from build123d import *

# Parameters (mm, degrees)
SKETCH_1_W          = 75
SKETCH_1_H          = 75
EXTRUDE_1_DEPTH     = 84
CHAMFER_1_SIZE      = 3
SKETCH_2_R          = 4.25
CUT_EXTRUDE_1_DEPTH = 85


with BuildPart() as part:
    # 草图1 → 凸台-拉伸1 (new body)
    with BuildSketch(Plane.XY):
        with Locations((37.5, -37.5)):
            Rectangle(SKETCH_1_W, SKETCH_1_H)
    extrude(amount=EXTRUDE_1_DEPTH)

    # 倒角1
    chamfer_1_edges = [part.edges().sort_by_distance(p)[0] for p in [
        (0, 0, 42),
        (75, 0, 42),
        (75, -75, 42),
        (0, -75, 42),
    ]]
    chamfer(chamfer_1_edges, length=CHAMFER_1_SIZE)

    # 草图2 → 切除-拉伸1 (cut, through all)
    with BuildSketch(Plane.XY.offset(84)):
        with Locations((7.5, -7.5)):
            Circle(SKETCH_2_R)
        with Locations((67.5, -7.5)):
            Circle(SKETCH_2_R)
        with Locations((67.5, -67.5)):
            Circle(SKETCH_2_R)
        with Locations((7.5, -67.5)):
            Circle(SKETCH_2_R)
    extrude(amount=-CUT_EXTRUDE_1_DEPTH, mode=Mode.SUBTRACT)


solid = part.part
Source: CAD feature listing. Evaluate the final solid. Frame: model axes, mm. Round coordinates to 2 decimals unless told otherwise and drop trailing zeros. Loops run counter-clockwise (first coordinate to the right, second up) from the corner with the lowest first, then second, coordinate; pieces in that order, holes last. Notation, with made-up numbers: (6.5, 68) -> (33.5, 68) arc R35 cw to (33.5, 100) -> close; hole circle Ø10 at (-32.5, 82). An arc over 180 degrees is marked (long way). Answer as a JSON object with one key per item and string values. Group by question number.
Q1. Ray query, line 1 (Y direction, x = 67.5, z = 62); line 2 (X direction, y = -7, z = 64); line 3 (X direction, y = -4, z = 25.5). Return the intervals inside material, ascending. Write a range as from..to.
Q2. Section query C-C (y = -7.5). Output: boundary loops of the cut face in (x, z).
Q3. Mould query, pull axis X, two halves, no side actions, for faces 1 (the cylindrical face through (71.426, -9.128, 42.588)), 2 (the flat face through (37, 0, 41)), 3 (the cylindrical face through (9.46, -71.27, 42.59)), 4 (the flat face through (74, -73, 41)). Classes: pulls with the +X half, pulls with the -X half, needs draft (parallel to the pull), parting line crosses it, or undercut.
Q4. Section query B-B (z = 27). Output: boundary loops of the cut face in (x, y), plus the area to 3 significant figures.
Q5. Section query A-A (x = 7.5). Output: boundary loops of the cut face in (y, z), plus the area to 3 significant figures.
Completed:
{
 "1": {"line 1": "-75..-71.75, -63.25..-11.75, -3.25..0", "line 2": "0..3.28, 11.72..63.28, 71.72..75", "line 3": "0..5.09, 9.91..65.09, 69.91..75"},
 "2": {"outline": "(0, 0) -> (3.25, 0) -> (3.25, 84) -> (0, 84) -> close; (11.75, 0) -> (63.25, 0) -> (63.25, 84) -> (11.75, 84) -> close; (71.75, 0) -> (75, 0) -> (75, 84) -> (71.75, 84) -> close"},
 "3": {"face 1": "undercut", "face 2": "needs draft", "face 3": "undercut", "face 4": "pulls with the +X half"},
 "4": {"outline": "(0, -72) -> (3, -75) -> (72, -75) -> (75, -72) -> (75, -3) -> (72, 0) -> (3, 0) -> (0, -3) -> close; hole circle Ø8.5 at (7.5, -67.5); hole circle Ø8.5 at (7.5, -7.5); hole circle Ø8.5 at (67.5, -67.5); hole circle Ø8.5 at (67.5, -7.5)", "area": "5,380 mm²"},
 "5": {"outline": "(-75, 0) -> (-71.75, 0) -> (-71.75, 84) -> (-75, 84) -> close; (-63.25, 0) -> (-11.75, 0) -> (-11.75, 84) -> (-63.25, 84) -> close; (-3.25, 0) -> (0, 0) -> (0, 84) -> (-3.25, 84) -> close", "area": "4,870 mm²"}
}
